CAD build for the part. Positions are in the model's coordinates, mm. Face numbers are marked on the shaded views. Coordinates: 2 decimals unless noted, no trailing zeros. Order: outer loops, then holes, each group sorted by start corner. A loop starts at its lowest first (then second) coordinate and runs counter-clockwise, first axis right, second up. Notation, with made-up numbers: M 23.5,56 L 42.5,56 A9 cw 42.5,69 Z; hole C 44,65.25 d1. An arc over 180 degrees is marked long. Write item = value, one per line.
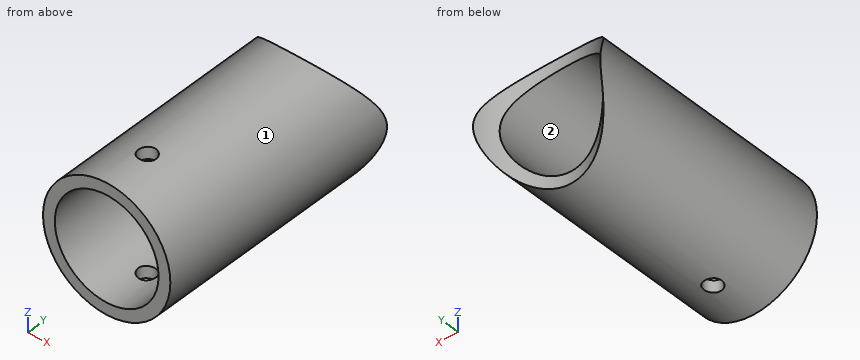
from build123d import *

# Parameters (mm, degrees)
F0_R     = 34.29
F0_R_2   = 27.94
F1_DEPTH = 76.2
F2_R     = 4.7625
F3_DEPTH = 38.1
F4_R     = 38.1
F5_DEPTH = 38.1


with BuildPart() as f1:
    # F0 (on Front) → F1 (new body, symmetric)
    with BuildSketch(Plane.XZ):
        Circle(F0_R)
        Circle(F0_R_2, mode=Mode.SUBTRACT)
    extrude(amount=F1_DEPTH, both=True)

    # F2 (on Top) → F3 (cut, symmetric)
    with BuildSketch(Plane.XY):
        with Locations((0, -50.8)):
            Circle(F2_R)
    extrude(amount=F3_DEPTH, both=True, mode=Mode.SUBTRACT)

    # F4 (on Top) → F5 (cut, symmetric)
    with BuildSketch(Plane.XY):
        with Locations((0, 76.2)):
            Circle(F4_R)
    extrude(amount=F5_DEPTH, both=True, mode=Mode.SUBTRACT)


solid = f1.part
(1) Slice it at A-A, the plane x = 0. Write the cut outline in (y, z), then the cut area to 3 significant figures.
Evaluation:
outline = M -76.2,-34.29 L -55.56,-34.29 L -55.56,-27.94 L -76.2,-27.94 Z; M -76.2,27.94 L -55.56,27.94 L -55.56,34.29 L -76.2,34.29 Z; M -46.04,-34.29 L 38.1,-34.29 L 38.1,-27.94 L -46.04,-27.94 Z; M -46.04,27.94 L 38.1,27.94 L 38.1,34.29 L -46.04,34.29 Z
area = 1,330 mm²
(2) Slice it at B-B, the plane z = 0. Write the cut outline in (x, y), then the cut area to 3 significant figures.
Evaluation:
outline = M -34.29,-76.2 L -27.94,-76.2 L -27.94,50.3 A38.1 cw -34.29,59.59 Z; M 27.94,-76.2 L 34.29,-76.2 L 34.29,59.59 A38.1 cw 27.94,50.3 Z
area = 1,660 mm²
(3) Slice it at D-D, the plane y = -26. Write the cut outline in (x, z), then the cut area to 3 significant figures.
Evaluation:
outline = C 0,0 d68.58; hole C 0,0 d55.88
area = 1,240 mm²
(4) Pull direction Z, two halves, no side cores. Call the marked faces 1 and 2: +Z half, -Z half, draft (parallel to the pull), parting line (faces both ways), or undercut.
Evaluation:
face_1 = parting line
face_2 = undercut
(5) Wall check: line 1 (Z direction, x = 0, y = -12); line 2 (Y direction, x = 0, z = -32). Give the ranges that are in metal, low to high. Write a range as from..to.
Evaluation:
line_1 = -34.29..-27.94, 27.94..34.29
line_2 = -76.2..-55.56, -46.04..38.1
(6) Pin check, flat tips, straight feed: pin 1 Ø3 at (y, z) = (-38.5, 18.5) entering from -X; pin 2 Ø3 at (x, y) = (24.5, -56) entering from -Z; pin 3 Ø1 at (x, y) = (21.5, 18) entering from -Z; pin 4 Ø11 at (x, y) = (0, -50.8) entering from -Z. Stop position of each tip, or through.
Evaluation:
pin_1 = -29.78
pin_2 = -25.43
pin_3 = -27.11
pin_4 = -34.29
(7) Slice it at C-C, the plane x = 10.5. Write the cut outline in (y, z), then the cut area to 3 significant figures.
Evaluation:
outline = M -76.2,-32.64 L 39.58,-32.64 L 39.58,-25.89 L -76.2,-25.89 Z; M -76.2,25.89 L 39.58,25.89 L 39.58,32.64 L -76.2,32.64 Z
area = 1,560 mm²
